```python
from build123d import *

# Parameters (mm, degrees)
SKETCH1_W           = 55.8
SKETCH1_H           = 9.3
BOSS_EXTRUDE1_DEPTH = 10


with BuildPart() as part:
    # Sketch1 → Boss-Extrude1 (new body)
    with BuildSketch(Plane(origin=(0, 0, 0), x_dir=(1, 0, 0), z_dir=(0, 1, 0))):
        with BuildLine():
            Line((0, 50), (177.8, 50))
            ThreePointArc((177.8, 50), (227.8, 0), (177.8, -50))
            Line((177.8, -50), (0, -50))
            ThreePointArc((0, -50), (-50, 0), (0, 50))
        make_face()
        with Locations((88.9, 40.35)):
            Rectangle(SKETCH1_W, SKETCH1_H, mode=Mode.SUBTRACT)
    extrude(amount=BOSS_EXTRUDE1_DEPTH)


solid = part.part
```
Work out the finished part from the listing and answer in its coordinate system (mm). A direction names the side the tool comes from. Round coordinates to 2 decimals unless told otherwise and drop trailing zeros. Write each loop counter-clockwise with the first axis right and the second up, starting at its lowest first coordinate (ties: lowest second). Pieces come first, ordered by that corner, then holes. Notation, with made-up numbers: (-30, -34.5) - (27, -34.5) arc R25 ccw to (27, -8.5) - close; hole circle Ø1 at (-38.75, 27). An arc over 180 degrees is marked (long way). Return JSON: item names as keys, results as strings. Group by question number.
Q1. The mould has two halves that part along Z. Classify faces 1 (the cylindrical face through (-49.988, 4.93, 1.099)), 2 (the flat face through (61, 5, -40)), 3 (the flat face through (90, 5, 50)): released by +Z, released by -Z, zero draft, split by the parting line, or undercut.
Q2. The part is cut by section C-C on z = -29.5. Write down the section's boundary in (x, y).
Q3. The part is cut by section B-B on x = -10. Write down the section's boundary in (y, z).
Q4. For faces 4 (the flat face through (116.8, 5, -40)), 5 (the flat face through (91, 10, -1)), determine the directions among +Z, -Z, +X, -X, +Y, -Y from which every point of the face is accessible in a straight line to the end or side of a thin tool.
Q5. The part is cut by section A-A on y = 6. Write down the section's boundary in (x, z).
Q6. Find the intervals of material crossed by L1, parallel to Z at x = 87.5, y = 2; L2, parallel to X at y = 1.75, z = -42; L3, parallel to X at y = 6.75, z = -8, in increasing order.
Q7. Each of these flat-tipped pins is pushed along its axis until it touches: pin 1 Ø3 at (y, z) = (3, -41.5) entering from +X; pin 2 Ø3 at (y, z) = (8.5, -31) entering from -X. Where does it stop, or does it pass through?
Solved:
{
 "1": {"face 1": "split by the parting line", "face 2": "undercut", "face 3": "released by +Z"},
 "2": {"outline": "(-40.37, 0) - (218.17, 0) - (218.17, 10) - (-40.37, 10) - close"},
 "3": {"outline": "(0, -48.99) - (10, -48.99) - (10, 48.99) - (0, 48.99) - close"},
 "4": {"face 4": "+Y, -Y", "face 5": "+Z, -Z, +X, -X, +Y"},
 "5": {"outline": "(0, -50) - (177.8, -50) arc R50 ccw to (177.8, 50) - (0, 50) arc R50 ccw to start; hole (61, -45) - (116.8, -45) - (116.8, -35.7) - (61, -35.7) - close"},
 "6": {"L1": "-50 to -45, -35.7 to 50", "L2": "-27.13 to 61, 116.8 to 204.93", "L3": "-49.36 to 227.16"},
 "7": {"pin 1": "x = 207.8", "pin 2": "x = -40.37"}
}
